Check sheet for the drawn part. Datum: minimum x, y, z corner. Units: mm. Round coordinates to 2 decimals unless told otherwise and drop trailing zeros. Order: outer loops, then holes, each group sorted by start corner. A loop starts at its lowest first (then second) coordinate and runs counter-clockwise, first axis right, second up.
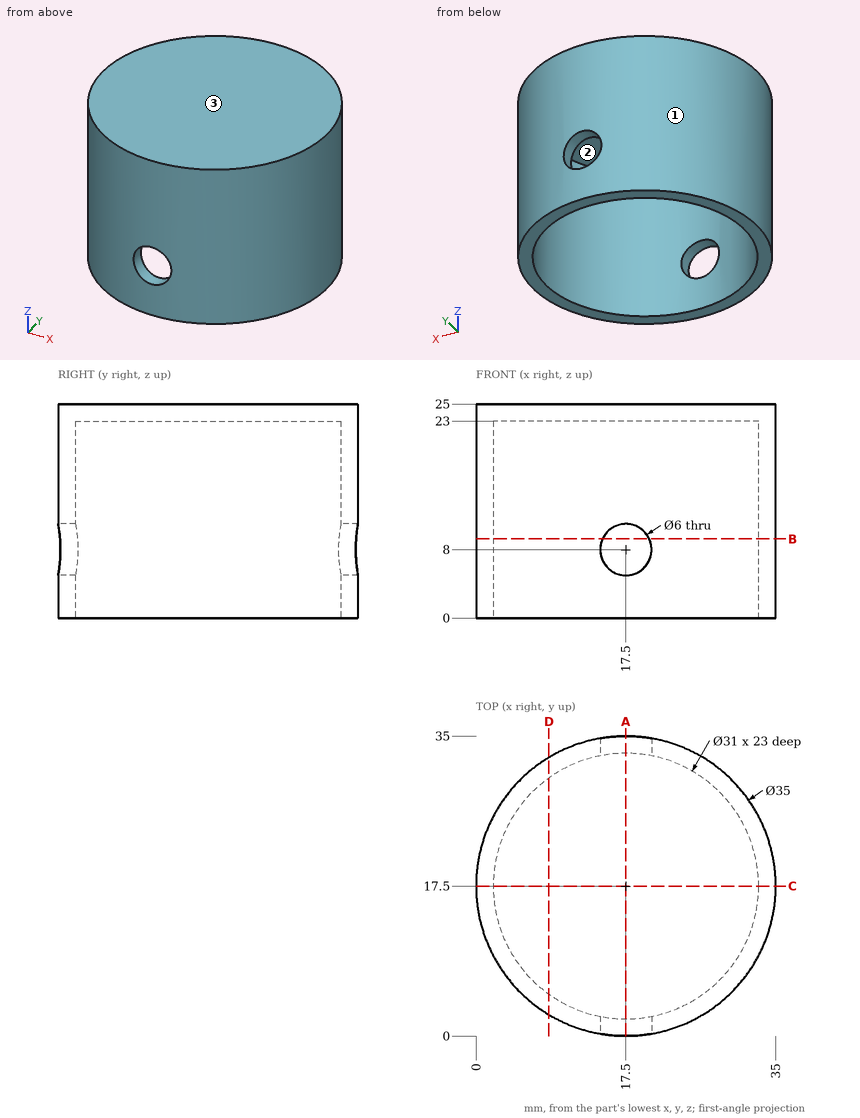
(1) Sectioned sample at B-B, the plane z = 9.25. Record the cut outline in (x, y), and give its area (3 significant figures).
Returned:
outline: (14.77, 0.21) - (14.77, 2.24) arc R15.5 cw to (14.77, 32.76) - (14.77, 34.79) arc R17.5 ccw to start; (20.23, 0.21) arc R17.5 ccw to (20.23, 34.79) - (20.23, 32.76) arc R15.5 cw to (20.23, 2.24) - close
area: 185 mm2
(2) Sectioned sample at C-C, the plane y = 17.5. Record the cut outline in (x, z), and give its area (3 significant figures).
Returned:
outline: (0, 0) - (2, 0) - (2, 23) - (33, 23) - (33, 0) - (35, 0) - (35, 25) - (0, 25) - close
area: 162 mm2
(3) Sectioned sample at D-D, the plane x = 8.5. Record the cut outline in (y, z), and give its area (3 significant figures).
Returned:
outline: (2.49, 0) - (4.88, 0) - (4.88, 23) - (30.12, 23) - (30.12, 0) - (32.51, 0) - (32.51, 25) - (2.49, 25) - close
area: 170 mm2
(4) Material ranges on line 1 (Z direction, x = 17.5, y = 34.45); line 2 (Z direction, x = 10, y = 9); line 3 (X direction, y = 10, z = 1), recorded low to high.
Returned:
line 1: z = 0 to 5, 11 to 25
line 2: z = 23 to 25
line 3: x = 1.69 to 3.94, 31.06 to 33.31
(5) Draft check along X on the marked faces 1, 2 and 3. Enter one of: released by +X, released by -X, zero draft, split by the parting line, or undercut.
Returned:
face 1: split by the parting line
face 2: undercut
face 3: zero draft
(6) Sectioned sample at A-A, the plane x = 17.5. Record the cut outline in (y, z), and give its area (3 significant figures).
Returned:
outline: (0, 0) - (2, 0) - (2, 5) - (0, 5) - close; (0, 11) - (2, 11) - (2, 23) - (33, 23) - (33, 11) - (35, 11) - (35, 25) - (0, 25) - close; (33, 0) - (35, 0) - (35, 5) - (33, 5) - close
area: 138 mm2
(7) Depth check by flat-ended pin: P1, Ø1, axis at x = 28, y = 24, coming from the -Z side; P2, Ø3, axis at y = 27.5, z = 20.5, coming from the -X side; P3, Ø4, axis at y = 21, z = 20.5, coming from the +X side. Enter the tip coordinate at first touch or a pass-through.
Returned:
P1: stops at z = 23
P2: stops at x = 2.2
P3: stops at x = 34.94
